The listing builds one solid part. Answer for the finished solid, in the listing's coordinates (mm). A direction names the side the tool comes from. Coordinates: 2 decimals unless noted, no trailing zeros. Return JSON: item names as keys, results as strings. Group by question number.
1. Which of the six approach directions +Z, -Z, +X, -X, +Y, -Y give full straight-line access (tool end or side, diameter ignored) to faces 1 (the face through (0, 0, 47.562)), 2 (the face through (0, 0, 77.066))?
2. Find the intervals of material crossed by line 1 along Z through (x, y) = (0, -8.2); line 2 along Z through (x, y) = (9.2, 0); line 3 along Y through (x, z) = (0, 37.25) (1 decimal), in increasing order.
3. Each of these flat-tipped pins is pushed along its axis until it touches: P1, Ø6, axis at y = 5.5, z = 66.5, coming from the +X side; P2, Ø4, axis at y = 0, z = 39.196, coming from the +X side (3 decimals); P3, Ø2, axis at y = 2.5, z = 36.5, coming from the -X side; P4, Ø6, axis at x = -1.5, z = 63, coming from the -Y side. Where does it stop, or does it pass through?
4. The mould has two halves that part along X. Classify faces 3 (the face through (-9.085, -2.861, 38.286)), 4 (the face through (-8.66, 0.07, 40.78)), 5 (the face through (0.07, -8.663, 31.578)): pulls with the +X half, pulls with the -X half, needs draft (parallel to the pull), parting line crosses it, or undercut.
```python
from build123d import *

# Parameters (mm, degrees)
SKETCH5_W               = 1.587499994
SKETCH5_H               = 54.90464
CUT_EXTRUDE5_DEPTH      = 79.234526804
CUT_EXTRUDE5_DEPTH_BACK = 79.234526804
SKETCH7_R               = 1.5875
CUT_EXTRUDE6_DEPTH      = 79.234526927
CUT_EXTRUDE6_DEPTH_BACK = 79.234526927
SKETCH6_R               = 1.5875
SKETCH10_R              = 7.9375
BOSS_EXTRUDE1_DEPTH     = 29.50464
CUT_EXTRUDE7_START      = 54.86908
SKETCH8_R               = 12.7
CUT_EXTRUDE7_DEPTH      = 25.4


with BuildPart() as part:
    # Sketch5 → Revolve2 (revolve)
    with BuildSketch(Plane(origin=(0, 0, 0), x_dir=(1, 0, 0), z_dir=(0, 1, 0)), mode=Mode.PRIVATE) as revolve2_sk:
        with Locations((8.731249997, -49.61382)):
            Rectangle(SKETCH5_W, SKETCH5_H)
    revolve(revolve2_sk.sketch.rotate(Axis((0, 0, 0), (0, 0, 1)), 180), axis=Axis((0, 0, 0), (0, 0, 1)))

    # Sketch7 → Cut-Extrude5 (cut, two sides: drawn at the far end of the back side and taken through both)
    with BuildSketch(Plane(origin=(0, 0, 0), x_dir=(0, 0, -1), z_dir=(1, 0, 0)).offset(-CUT_EXTRUDE5_DEPTH_BACK)):
        with Locations((-39.195999993, 0)):
            Circle(SKETCH7_R)
    extrude(amount=CUT_EXTRUDE5_DEPTH + CUT_EXTRUDE5_DEPTH_BACK, mode=Mode.SUBTRACT)

    # Sketch6 → Cut-Extrude6 (cut, two sides: drawn at the far end of the back side and taken through both)
    with BuildSketch(Plane(origin=(0, 0, 0), x_dir=(1, 0, 0), z_dir=(0, 1, 0)).offset(-CUT_EXTRUDE6_DEPTH_BACK)):
        with Locations(Location((1e-09, -33.163499999, 0), (0, 0, 269.999999955))):
            Circle(SKETCH6_R)
    extrude(amount=CUT_EXTRUDE6_DEPTH + CUT_EXTRUDE6_DEPTH_BACK, mode=Mode.SUBTRACT)

    # Sketch10 → Boss-Extrude1 (add)
    with BuildSketch(Plane(origin=(0, 0, 47.5615), x_dir=(-1, 0, 0), z_dir=(0, 0, -1))):
        Circle(SKETCH10_R)
    extrude(amount=-BOSS_EXTRUDE1_DEPTH)

    # Sketch8 → Cut-Extrude7 (cut)
    with BuildSketch(Plane.XY.offset(CUT_EXTRUDE7_START)):
        Circle(SKETCH8_R)
        Polygon((9.235721046, -0.808020891), (8.681700155, -0.254), (8.681700155, 0.254), (9.235721046, 0.808020891), (8.593912259, 1.257420242), (8.505698985, 1.75770258), (8.955098336, 2.399511367), (8.245002688, 2.730634406), (8.071256455, 3.207998257), (8.402379494, 3.918093905), (7.645572882, 4.120879625), (7.391572882, 4.56082053), (7.594358603, 5.317627141), (6.813836213, 5.385914002), (6.487300108, 5.775064579), (6.555586968, 6.555586968), (5.775064579, 6.487300108), (5.385914002, 6.813836213), (5.317627141, 7.594358603), (4.56082053, 7.391572882), (4.120879625, 7.645572882), (3.918093905, 8.402379494), (3.207998257, 8.071256455), (2.730634406, 8.245002688), (2.399511367, 8.955098336), (1.75770258, 8.505698985), (1.257420242, 8.593912259), (0.808020891, 9.235721046), (0.254, 8.681700155), (-0.254, 8.681700155), (-0.808020891, 9.235721046), (-1.257420242, 8.593912259), (-1.75770258, 8.505698985), (-2.399511367, 8.955098336), (-2.730634406, 8.245002688), (-3.207998257, 8.071256455), (-3.918093905, 8.402379494), (-4.120879625, 7.645572882), (-4.56082053, 7.391572882), (-5.317627141, 7.594358603), (-5.385914002, 6.813836213), (-5.775064579, 6.487300108), (-6.555586968, 6.555586968), (-6.487300108, 5.775064579), (-6.813836213, 5.385914002), (-7.594358603, 5.317627141), (-7.391572882, 4.56082053), (-7.645572882, 4.120879625), (-8.402379494, 3.918093905), (-8.071256455, 3.207998257), (-8.245002688, 2.730634406), (-8.955098336, 2.399511367), (-8.505698985, 1.75770258), (-8.593912259, 1.257420242), (-9.235721046, 0.808020891), (-8.681700155, 0.254), (-8.681700155, -0.254), (-9.235721046, -0.808020891), (-8.593912259, -1.257420242), (-8.505698985, -1.75770258), (-8.955098336, -2.399511367), (-8.245002688, -2.730634406), (-8.071256455, -3.207998257), (-8.402379494, -3.918093905), (-7.645572882, -4.120879625), (-7.391572882, -4.56082053), (-7.594358603, -5.317627141), (-6.813836213, -5.385914002), (-6.487300108, -5.775064579), (-6.555586968, -6.555586968), (-5.775064579, -6.487300108), (-5.385914002, -6.813836213), (-5.317627141, -7.594358603), (-4.56082053, -7.391572882), (-4.120879625, -7.645572882), (-3.918093905, -8.402379494), (-3.207998257, -8.071256455), (-2.730634406, -8.245002688), (-2.399511367, -8.955098336), (-1.75770258, -8.505698985), (-1.257420242, -8.593912259), (-0.808020891, -9.235721046), (-0.254, -8.681700155), (0.254, -8.681700155), (0.808020891, -9.235721046), (1.257420242, -8.593912259), (1.75770258, -8.505698985), (2.399511367, -8.955098336), (2.730634406, -8.245002688), (3.207998257, -8.071256455), (3.918093905, -8.402379494), (4.120879625, -7.645572882), (4.56082053, -7.391572882), (5.317627141, -7.594358603), (5.385914002, -6.813836213), (5.775064579, -6.487300108), (6.555586968, -6.555586968), (6.487300108, -5.775064579), (6.813836213, -5.385914002), (7.594358603, -5.317627141), (7.391572882, -4.56082053), (7.645572882, -4.120879625), (8.402379494, -3.918093905), (8.071256455, -3.207998257), (8.245002688, -2.730634406), (8.955098336, -2.399511367), (8.505698985, -1.75770258), (8.593912259, -1.257420242), align=None, mode=Mode.SUBTRACT)
    extrude(amount=CUT_EXTRUDE7_DEPTH, mode=Mode.SUBTRACT)


solid = part.part
```
The answers:
{
 "1": {"face 1": "-Z", "face 2": "+Z, +X, -X, +Y, -Y"},
 "2": {"line 1": "z = 22.16 to 31.58, 34.75 to 77.07", "line 2": "z = 22.16 to 37.61, 40.78 to 54.87", "line 3": "y = -9.5 to -7.9, 7.9 to 9.5"},
 "3": {"P1": "stops at x = 8.74", "P2": "stops at x = 9.525", "P3": "stops at x = -9.41", "P4": "stops at y = -9.24"},
 "4": {"face 3": "parting line crosses it", "face 4": "needs draft", "face 5": "undercut"}
}
